Autodesk Inventor part; units mm, degrees
ref_plane "YZ Plane" through (0, 0, 0) normal (1, 0, 0) x (0, 1, 0)
ref_plane "XZ Plane" through (0, 0, 0) normal (0, 1, 0) x (-1, 0, 0)
ref_plane "XY Plane" through (0, 0, 0) normal (0, 0, 1) x (1, 0, 0)
sketch "草图1" plane through (0, 0, 0) normal (1, 0, 0) x (0, 1, 0)
  line L0 (162.5, 180) -> (-162.5, 180)
  line L1 (-162.5, 180) -> (-162.5, -180)
  line L2 (-162.5, -180) -> (162.5, -180)
  line L3 (162.5, -180) -> (162.5, 180)
  line L4 (162.5, 180) -> (-162.5, -180) construction
  line L5 (-162.5, 180) -> (162.5, -180) construction
  circle A0 centre (0, 0) radius 20
  line L6 (-10, 200) -> (10, 200)
  line L7 (10, 200) -> (10, 180)
  line L8 (10, 180) -> (-10, 180)
  line L9 (-10, 180) -> (-10, 200)
  line L10 (-10, 200) -> (10, 180) construction
  line L11 (10, 200) -> (-10, 180) construction
  point P0 (0, 190)
  point P1 (0, 190)
  dimension "d0" = 325
  dimension "d1" = 360
  dimension "d2" = 40
  dimension "d54" = 20
  dimension "d55" = 20
extrude "拉伸1" add sketch "草图1" along normal blind 8
chamfer "倒角1" distance 2 angle 45 4 edges at (4, 162.5, 180) (4, 162.5, -180) (4, -162.5, 180) (4, -162.5, -180)
sketch "草图2" plane through (8, 0, 0) normal (1, 0, 0) x (0, 0, -1)
  line L0 (178, 162.5) -> (-178, 162.5)
  line L1 (-180, 160.5) -> (-180, -160.5)
  line L2 (180, -160.5) -> (180, 160.5)
  line L3 (-178, -162.5) -> (178, -162.5)
  point P0 (0, 0)
  point P1 (148, 71)
  point P2 (148, 47)
  point P3 (172, 71)
  point P4 (172, 47)
  point P5 (172, -71)
  point P6 (172, -47)
  point P7 (148, -71)
  point P8 (148, -47)
  dimension "d8" = 91.5
  dimension "d12" = 24
  dimension "d15" = 24
  dimension "d20" = 118
  dimension "d25" = 94
  dimension "d26" = 142
  dimension "d27" = 352
  dimension "d50" = 8
  dimension "d51" = 91.5
hole "孔1" at (8, 71, -148) at (8, 47, -148) at (8, 71, -172) at (8, 47, -172) at (8, -71, -172) at (8, -47, -172) at (8, -71, -148) at (8, -47, -148) direction (-1, 0, 0) diameter 4.917 end through all
sketch "草图3" plane through (8, 0, 0) normal (1, 0, 0) x (0, 0, -1)
  line L0 (0, 0) -> (-35.3553, 35.3553) construction
  line L1 (-178, -162.5) -> (178, -162.5)
  line L2 (0, 0) -> (-35.3553, -35.3553) construction
  line L3 (0, 0) -> (35.3553, -35.3553) construction
  line L4 (0, 0) -> (35.3553, 35.3553) construction
  dimension "d35" = 45
  dimension "d36" = 50
  dimension "d39" = 360
hole "孔2" at (8, 35.3553, 35.3553) at (8, -35.3553, 35.3553) at (8, -35.3553, -35.3553) at (8, 35.3553, -35.3553) direction (-1, 0, 0) diameter 6.647 end through all
chamfer "倒角2" distance 2 angle 45 2 edges at (4, 10, 200) (4, -10, 200)
properties part number "CTQCX300.2-1门板" material "钢板B-8/SUS304"
Geometry: final body of the model. Coordinates: model frame, mm. A direction names the side the tool comes from. Round coordinates to 2 decimals unless told otherwise and drop trailing zeros. Order: outer loops, then holes, each group sorted by start corner. A loop starts at its lowest first (then second) coordinate and runs counter-clockwise, first axis right, second up. Notation, with made-up numbers: (88, 11) -> (93, 11) arc R34 cw to (93, 48) -> close; hole circle Ø7 at (59.25, 5.25). An arc over 180 degrees is marked (long way). Use one line per item in the form item = value.
(1) Draft query along Y for faces 3 (the face through (4, -84, 180)), 4 (the face through (3.944, -4.336, 19.524)), 5 (the face through (4, -10, 189)). Return one class per face: pulls with the +Y half, pulls with the -Y half, needs draft (parallel to the pull), parting line crosses it, or undercut.
Results list:
face_3 = needs draft
face_4 = undercut
face_5 = pulls with the -Y half
(2) Section B-B on x = 6.25. Count the separate pieces of the cut face and the enclosed holes in it, and give its area (3 significant figures).
Results list:
separate_pieces = 1
enclosed_holes = 13
area = 116,000 mm^2
(3) First-contact query: pin 1 Ø4 at (x, y) = (2.5, 69) entering from +Z; pin 2 Ø3 at (y, z) = (-71, -148) entering from +X; pin 3 Ø2.5 at (x, z) = (5, 192) entering from -Y. Flat tips, straight axial feed; report the tip coordinate or a pass-through.
Results list:
pin_1 = 180
pin_2 = through
pin_3 = -10
(4) Section A-A on y = 0. Return loops of the section in (x, z).
Results list:
outline = (0, -180) -> (8, -180) -> (8, -20) -> (0, -20) -> close; (0, 20) -> (8, 20) -> (8, 200) -> (0, 200) -> close
(5) Ray query, probe 1 along Y at (x, z) = (3.5, -172); probe 2 along Z at (x, y) = (4, -47); probe 3 along Y at (x, z) = (6.75, -0.5). Return the intervals inside material, ascending. Write a range as [from, to].
Results list:
probe_1 = [-162.5, -73.46], [-68.54, -49.46], [-44.54, 44.54], [49.46, 68.54], [73.46, 162.5]
probe_2 = [-180, -174.46], [-169.54, -150.46], [-145.54, 180]
probe_3 = [-162.5, -19.99], [19.99, 162.5]
(6) Section C-C on y = -114.5. Return loops of the section in (x, z).
Results list:
outline = (0, -180) -> (8, -180) -> (8, 180) -> (0, 180) -> close
(7) Access query for faces 1 (the face through (4, 10, 189)), 2 (the face through (0, -2, -30)). Directions: +Z, -Z, +X, -X, +Y, -Y. A direction counts if a zero-diameter tool reaches every point of the face in a straight line with its end or side. Return the directions, or none.
Results list:
face_1 = +Z, +X, -X, +Y
face_2 = +Z, -Z, -X, +Y, -Y
